```python
from build123d import *

# Parameters (mm, degrees)
SKETCH1_W           = 63.5
SKETCH1_H           = 63.5
BOSS_EXTRUDE1_DEPTH = 1.27
SKETCH2_R           = 1.905
CUT_EXTRUDE1_DEPTH  = 1.27
SKETCH3_W           = 44.45
SKETCH3_H           = 19.05
CUT_EXTRUDE2_DEPTH  = 1.27
SKETCH4_R           = 0.73025
BOSS_EXTRUDE2_DEPTH = 3.81
CUT_EXTRUDE3_REACH  = 5.81
SKETCH5_W           = 26.162
SKETCH5_H           = 19.685


with BuildPart() as part:
    # Sketch1 → Boss-Extrude1 (new body)
    with BuildSketch(Plane(origin=(0, 0, 0), x_dir=(1, 0, 0), z_dir=(0, 1, 0))):
        Rectangle(SKETCH1_W, SKETCH1_H)
    extrude(amount=BOSS_EXTRUDE1_DEPTH)

    # Sketch2 → Cut-Extrude1 (cut)
    with BuildSketch(Plane(origin=(0, 1.27, 0), x_dir=(1, 0, 0), z_dir=(0, 1, 0))):
        with Locations((27.0129, 7.62)):
            Circle(SKETCH2_R)
        with Locations((25.9715, 26.67)):
            Circle(SKETCH2_R)
        with Locations((-27.0129, 7.62)):
            Circle(SKETCH2_R)
        with Locations((-25.9715, 26.67)):
            Circle(SKETCH2_R)
    extrude(amount=-CUT_EXTRUDE1_DEPTH, mode=Mode.SUBTRACT)

    # Sketch3 → Cut-Extrude2 (cut)
    with BuildSketch(Plane(origin=(0, 1.27, 0), x_dir=(1, 0, 0), z_dir=(0, 1, 0))):
        with Locations((0, 15.875)):
            Rectangle(SKETCH3_W, SKETCH3_H)
    extrude(amount=-CUT_EXTRUDE2_DEPTH, mode=Mode.SUBTRACT)

    # Sketch4 → Boss-Extrude2 (add)
    with BuildSketch(Plane(origin=(0, 1.27, 0), x_dir=(1, 0, 0), z_dir=(0, 1, 0))):
        with Locations((-15.748, -7.3025)):
            Circle(SKETCH4_R)
        with Locations((15.748, -19.3167)):
            Circle(SKETCH4_R)
    extrude(amount=-BOSS_EXTRUDE2_DEPTH)

    # Sketch5 → Cut-Extrude3 (cut, up to next)
    with BuildSketch(Plane(origin=(0, 1.27, 0), x_dir=(1, 0, 0), z_dir=(0, 1, 0)), mode=Mode.PRIVATE) as cut_extrude3_sk1:
        with Locations((0, -15.875)):
            Rectangle(SKETCH5_W, SKETCH5_H)
    cut_extrude3_tool1 = extrude(cut_extrude3_sk1.sketch, amount=-CUT_EXTRUDE3_REACH, mode=Mode.PRIVATE) & part.part
    add(cut_extrude3_tool1.solids().sort_by_distance((0, 1.27, 15.875))[0], mode=Mode.SUBTRACT)


solid = part.part
```
Can you work these out from the model? Positions are in its coordinate system, mm. A direction names the side the tool comes from. Round coordinates to 2 decimals unless told otherwise and drop trailing zeros. Order: outer loops, then holes, each group sorted by start corner. A loop starts at its lowest first (then second) coordinate and runs counter-clockwise, first axis right, second up.
(1) If I drill on L1, parallel to X at y = 0.4, z = -7.62 (3 decimals); L2, parallel to X at y = 0.95, z = -26.67; L3, parallel to Z at x = 21, y = 0.45, over which ranges is the centre line in solid material (lowest first)?
Results are:
L1: x = -31.75 to -28.918, -25.108 to -22.225, 22.225 to 25.108, 28.918 to 31.75
L2: x = -31.75 to -27.88, -24.07 to 24.07, 27.88 to 31.75
L3: z = -31.75 to -25.4, -6.35 to 31.75
(2) We'd pull the mould along X, two halves only. Please class faces 3 (the face through (-15.073, -1.252, 7.582)), 4 (the face through (0, 1.27, 0)), 5 (the face through (-27.875, 0.644, -26.754)), 6 (the face through (-27.26, 0.64, -9.51)): +X half, -X half, draft (parallel to the pull), parting line (faces both ways), or undercut.
Results are:
face 3: parting line
face 4: draft
face 5: undercut
face 6: undercut
(3) If we section it at A-A (x = -18.5): Please give me the cut outline in (y, z).
Results are:
outline: (0, -31.75) - (1.27, -31.75) - (1.27, -25.4) - (0, -25.4) - close; (0, -6.35) - (1.27, -6.35) - (1.27, 31.75) - (0, 31.75) - close
(4) If we section it at B-B (z = 22): Please give me the cut outline in (x, y).
Results are:
outline: (-31.75, 0) - (-13.08, 0) - (-13.08, 1.27) - (-31.75, 1.27) - close; (13.08, 0) - (31.75, 0) - (31.75, 1.27) - (13.08, 1.27) - close
(5) I'm going to push a flat-ended pin straight in: pin 1 (5 mm diameter, centred on x = -27.01, z = -7.62, fed in from -Y). Where does the tip first touch, or does it pass through?
Results are:
pin 1: stops at y = 0
(6) If we section it at C-C (x = 0.5): Please give me the cut outline in (y, z).
Results are:
outline: (0, -31.75) - (1.27, -31.75) - (1.27, -25.4) - (0, -25.4) - close; (0, -6.35) - (1.27, -6.35) - (1.27, 6.03) - (0, 6.03) - close; (0, 25.72) - (1.27, 25.72) - (1.27, 31.75) - (0, 31.75) - close
(7) If we section it at D-D (z = -26.67): Please give me the cut outline in (x, y).
Results are:
outline: (-31.75, 0) - (-27.88, 0) - (-27.88, 1.27) - (-31.75, 1.27) - close; (-24.07, 0) - (24.07, 0) - (24.07, 1.27) - (-24.07, 1.27) - close; (27.88, 0) - (31.75, 0) - (31.75, 1.27) - (27.88, 1.27) - close
(8) On a 3-axis mill with a long thin cutter (end or side, diameter ignored), from which of +Z, -Z, +X, -X, +Y, -Y can I reach the whole of each face in a straight line? I mean faces 1 (the face through (24.07, 0.64, -26.75)), 2 (the face through (15.02, -1.25, 19.28)). Say none if no direction works.
Results are:
face 1: +Y, -Y
face 2: -Y
